from build123d import *

# Parameters (mm, degrees)
F0_W     = 50.8
F0_H     = 50.8
F1_DEPTH = 50.8
F2_R     = 12.7
F3_DEPTH = 50.8
F4_W     = 15.6972
F4_H     = 13.5128
F5_DEPTH = 5.842
F6_R     = 7.577209
F7_DEPTH = 5.08


with BuildPart() as f1:
    # F0 (on Front) → F1 (new body)
    with BuildSketch(Plane.XZ):
        with Locations((-25.4, 25.4)):
            Rectangle(F0_W, F0_H)
    extrude(amount=F1_DEPTH)

    # F2 (on face) → F3 (cut)
    with BuildSketch(Plane.XZ.offset(50.8)):
        with Locations((-25.4, 25.4)):
            Circle(F2_R)
    extrude(amount=-F3_DEPTH, mode=Mode.SUBTRACT)

    # F4 (on face) → F5 (join)
    with BuildSketch(Plane(origin=(-50.8, 0, 0), x_dir=(0, -1, 0), z_dir=(-1, 0, 0))):
        with Locations((27.126858, 23.556107)):
            Rectangle(F4_W, F4_H)
    extrude(amount=F5_DEPTH)

    # F6 (on face) → F7 (join)
    with BuildSketch(Plane.XY.offset(50.8)):
        with Locations((-25.4, -25.4)):
            Circle(F6_R)
    extrude(amount=F7_DEPTH)


solid = f1.part
Work out the finished part from the listing and answer in its coordinate system (mm). A direction names the side the tool comes from. Round coordinates to 2 decimals unless told otherwise and drop trailing zeros. Order: outer loops, then holes, each group sorted by start corner. A loop starts at its lowest first (then second) coordinate and runs counter-clockwise, first axis right, second up. Notation, with made-up numbers: M -26.75,51.25 L 5.25,51.25 A13 cw 5.25,55.25 Z; hole C 88.25,50.25 d6. An arc over 180 degrees is marked long. Put each result on its own line as item: value. Start each with the question number.
Q1. For a pull along X with two mould halves and no side action, classify faces 1 (the flat face through (-31, -50.8, 37)), 2 (the cylindrical face through (-30.985, -20.279, 53.304)), 3 (the cylindrical face through (-18.573, -25.756, 36.109)) as pulls with the +X half, pulls with the -X half, needs draft (parallel to the pull), parting line crosses it, or undercut.
Q2. Flat-ended cylindrical pins translate along their axes: pin 1 (1.8 mm diameter, centred on x = -54, z = 21.5, fed in from +Y); pin 2 (3 mm diameter, centred on x = -52.5, z = 21.5, fed in from -Y); pin 3 (3 mm diameter, centred on x = -52.5, y = -29.5, fed in from -Z). Find the tip coordinate at first contact, or state that the pin passes through.
Q3. Section C-C, the plane x = -16.5 is taken. Write down the section's boundary in (y, z).
Q4. A tool of negligible diameter and unlimited length cuts with its end or side. For faces 4 (the flat face through (-54, -34.975, 23)), 5 (the flat face through (-54, -19.278, 23)), 6 (the flat face through (-54, -27, 16.8)), 7 (the flat face through (-54, -27, 30.313)), from which of +Z, -Z, +X, -X, +Y, -Y can it reach the whole face along a straight path? Write none if from no direction.
Q5. Section A-A, the plane z = 25.4 is taken. Write down the section's boundary in (x, y).
Q6. Straight lines are drawn through the part: L1, parallel to X at y = -33, z = 25; L2, parallel to X at y = -14, z = 49.5; L3, parallel to Z at x = -49.5, y = -2. For each, find the intervals that lie inside material, in ascending order. Write a range as [from, to].
Q7. Section D-D, the plane y = -36.5 is taken. Write down the section's boundary in (x, z).
Q8. Section B-B, the plane y = -25.4 is taken. Write down the section's boundary in (x, z), and give its area (3 significant figures).
Findings below:
1. face 1: needs draft
1. face 2: parting line crosses it
1. face 3: undercut
2. pin 1: stops at y = -19.28
2. pin 2: stops at y = -34.98
2. pin 3: stops at z = 16.8
3. outline: M -50.8,0 L 0,0 L 0,16.34 L -50.8,16.34 Z; M -50.8,34.46 L 0,34.46 L 0,50.8 L -50.8,50.8 Z
4. face 4: +Z, -Z, -X, -Y
4. face 5: +Z, -Z, -X, +Y
4. face 6: -Z, -X, +Y, -Y
4. face 7: +Z, -X, +Y, -Y
5. outline: M -56.64,-34.98 L -50.8,-34.98 L -50.8,-50.8 L -38.1,-50.8 L -38.1,0 L -50.8,0 L -50.8,-19.28 L -56.64,-19.28 Z; M -12.7,-50.8 L 0,-50.8 L 0,0 L -12.7,0 Z
6. L1: x = [-56.64, -38.09], [-12.71, 0]
6. L2: x = [-50.8, 0]
6. L3: z = [0, 50.8]
7. outline: M -50.8,0 L 0,0 L 0,50.8 L -50.8,50.8 Z; hole C -25.4,25.4 d25.4
8. outline: M -56.64,16.8 L -50.8,16.8 L -50.8,0 L 0,0 L 0,50.8 L -17.82,50.8 L -17.82,55.88 L -32.98,55.88 L -32.98,50.8 L -50.8,50.8 L -50.8,30.31 L -56.64,30.31 Z; hole C -25.4,25.4 d25.4
8. area: 2,230 mm^2
